Here's how the part is built. I have some questions about the finished solid (model axes, mm). Round coordinates to 2 decimals unless told otherwise and drop trailing zeros. Loops run counter-clockwise (first coordinate to the right, second up) from the corner with the lowest first, then second, coordinate; pieces in that order, holes last. Notation, with made-up numbers: M 75,-36 L 112,-36 A4 cw 112,-30 Z; hole C -35,13.5 d11. An arc over 180 degrees is marked long. Put each result on its own line as item: value. Start each with the question number.
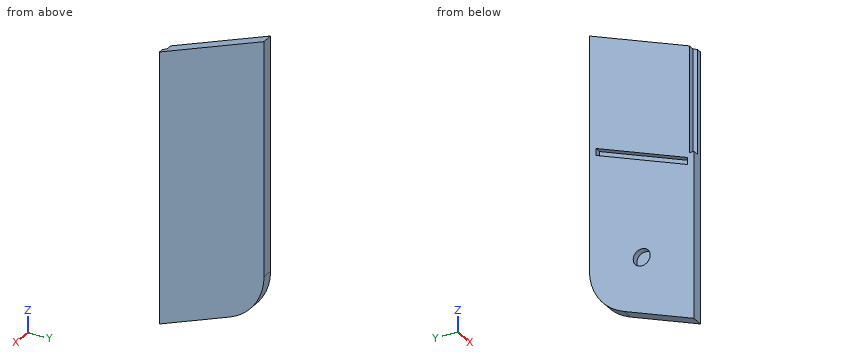
```python
from build123d import *

# Parameters (mm, degrees)
F1_DEPTH = 9
F2_R     = 6.5
F3_DEPTH = 5
F5_DEPTH = 5
F7_DEPTH = 5


with BuildPart() as f1:
    # F0 (on Right) → F1 (new body)
    with BuildSketch(Plane.YZ):
        with BuildLine():
            Line((80, 29.117619), (0, 0))
            Line((0, 0), (0, -207.12592))
            Line((0, -207.12592), (53.680806, -187.587705))
            ThreePointArc((53.680806, -187.587705), (72.766082, -172.943057), (80, -150))
            Line((80, -150), (80, 29.117619))
        make_face()
    extrude(amount=F1_DEPTH)

    # F2 (on face) → F3 (cut)
    with BuildSketch(Plane(origin=(0, 0, 0), x_dir=(0, -1, 0), z_dir=(-1, 0, 0))):
        with Locations((-40, -150)):
            Circle(F2_R)
    extrude(amount=-F3_DEPTH, mode=Mode.SUBTRACT)

    # F4 (on face) → F5 (cut)
    with BuildSketch(Plane(origin=(0, 0, 0), x_dir=(0, -1, 0), z_dir=(-1, 0, 0))):
        Polygon((-5, -88.635259), (-5, -83.314371), (-75, -57.836454), (-75, -63.157343), align=None)
    extrude(amount=-F5_DEPTH, mode=Mode.SUBTRACT)

    # F6 (on face) → F7 (cut)
    with BuildSketch(Plane(origin=(0, 0, 0), x_dir=(0, -1, 0), z_dir=(-1, 0, 0))):
        Polygon((0, 0), (-3.5, 1.273896), (-3.5, -80), (0, -80), align=None)
    extrude(amount=-F7_DEPTH, mode=Mode.SUBTRACT)


solid = f1.part
```
1) Suppose I cut it at C-C (z = -18). Write out the boundary of the cut face in (x, y).
2) Suppose I cut it at B-B (y = 71). Write out the boundary of the cut face in (x, z).
3) If I drill on probe 1 along Z at (x, y) = (2.8, 40); probe 2 along X at (y, z) = (34, -76.5); probe 3 along Y at (x, z) = (1.25, -14.5), over which ranges is the centre line in solid material (lowest first)? Write a range as from..to.
4) Suppose I cut it at D-D (y = 35.5). Write out the boundary of the cut face in (x, z), plus the area to 3 significant figures.
5) I'm going to push flat-ended pins straight in: P1, Ø5, axis at x = 7.5, y = 37.5, coming from the +Z side; P2, Ø5, axis at x = 7, y = 12, coming from the -Z side; P3, Ø1.5, axis at x = 3.5, z = -6.5, coming from the -Y side. Where does each tip first touch, or does it pass through?
6) Suppose I cut it at A-A (x = 2). Write out the boundary of the cut face in (y, z), plus the area to 3 significant figures.
Results are:
1. outline: M 0,3.5 L 5,3.5 L 5,0 L 9,0 L 9,80 L 0,80 Z
2. outline: M 0,-175.28 L 9,-175.28 L 9,25.84 L 0,25.84 L 0,-59.29 L 5,-59.29 L 5,-64.61 L 0,-64.61 Z
3. probe 1: -192.57..-156.5, -143.5..-75.9, -70.58..14.56
3. probe 2: 5..9
3. probe 3: 3.5..80
4. outline: M 0,-194.2 L 9,-194.2 L 9,12.92 L 0,12.92 L 0,-72.21 L 5,-72.21 L 5,-77.53 L 0,-77.53 L 0,-145.31 L 5,-145.31 L 5,-154.69 L 0,-154.69 Z
4. area: 1,790 mm²
5. P1: z = 14.56
5. P2: z = -203.67
5. P3: y = 3.5
6. outline: M 0,-207.13 L 53.68,-187.59 A40 ccw 80,-150 L 80,29.12 L 3.5,1.27 L 3.5,-80 L 0,-80 Z; hole M 5,-88.64 L 75,-63.16 L 75,-57.84 L 5,-83.31 Z; hole C 40,-150 d13
6. area: 15,600 mm²
